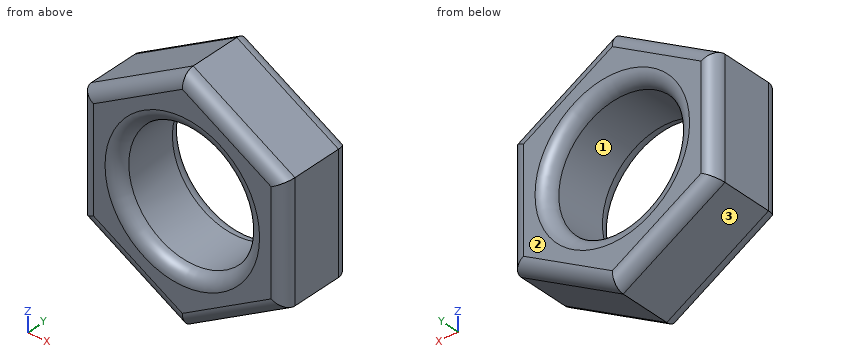
Autodesk Inventor part; units mm, degrees
ref_plane "YZ Plane" through (0, 0, 0) normal (1, 0, 0) x (0, 1, 0)
ref_plane "XZ Plane" through (0, 0, 0) normal (0, 1, 0) x (-1, 0, 0)
ref_plane "XY Plane" through (0, 0, 0) normal (0, 0, 1) x (1, 0, 0)
sketch "Sketch1" plane through (0, 0, 0) normal (0, 1, 0) x (-1, 0, 0)
  line L0 (3.95, -2.2805) -> (0, -4.5611)
  line L1 (0, -4.5611) -> (-3.95, -2.2805)
  line L2 (-3.95, -2.2805) -> (-3.95, 2.2805)
  line L3 (-3.95, 2.2805) -> (0, 4.5611)
  line L4 (0, 4.5611) -> (3.95, 2.2805)
  line L5 (3.95, 2.2805) -> (3.95, -2.2805)
  circle A0 centre (0, 0) radius 2.5
  dimension "d0" = 3.95
  dimension "d1" = 5
extrude "Extrusion1" add sketch "Sketch1" along normal blind 3
fillet "Fillet1" radius 0.5 14 edges at (3.95, 3, 0) (1.975, 3, -3.4208) (-1.975, 3, -3.4208) (-3.95, 3, 0) (-1.975, 3, 3.4208) (1.975, 3, 3.4208) (3.95, 0, 0) (1.975, 0, 3.4208) (-1.975, 0, 3.4208) (-3.95, 0, 0) (-1.975, 0, -3.4208) (1.975, 0, -3.4208) (2.5, 0, 0) (2.5, 3, 0)
thread "Thread1"
properties part number "M5 Nut Silver"
Geometry: final body of the model. Coordinates: model frame, mm. Face numbers are marked on the shaded views. Coordinates: 2 decimals unless noted, no trailing zeros. Order: outer loops, then holes, each group sorted by start corner. A loop starts at its lowest first (then second) coordinate and runs counter-clockwise, first axis right, second up.
Item 1: Section query B-B (y = 0.85). Output: boundary loops of the cut face in (x, z).
Answer:
outline: (-3.95, -2.28) - (0, -4.56) - (3.95, -2.28) - (3.95, 2.28) - (0, 4.56) - (-3.95, 2.28) - close; hole circle Ø5 at (0, 0)
Item 2: Material intervals for line 1 along Z through (x, y) = (-0.25, 1.2); line 2 along Z through (x, y) = (-0.75, 0.25); line 3 along X through (y, z) = (0.5, -1), sorted ascending.
Answer:
line 1: z = -4.42 to -2.49, 2.49 to 4.42
line 2: z = -4.05 to -2.45, 2.45 to 4.05
line 3: x = -3.95 to -2.29, 2.29 to 3.95
Item 3: Section query A-A (z = 0). Output: boundary loops of the cut face in (x, y), then the cut area to 3 significant figures.
Answer:
outline: (-3.95, 0.5) arc R0.5 ccw to (-3.45, 0) - (-3, 0) arc R0.5 ccw to (-2.5, 0.5) - (-2.5, 2.5) arc R0.5 ccw to (-3, 3) - (-3.45, 3) arc R0.5 ccw to (-3.95, 2.5) - close; (2.5, 0.5) arc R0.5 ccw to (3, 0) - (3.45, 0) arc R0.5 ccw to (3.95, 0.5) - (3.95, 2.5) arc R0.5 ccw to (3.45, 3) - (3, 3) arc R0.5 ccw to (2.5, 2.5) - close
area: 8.27 mm2
Item 4: Contact query for a flat-ended pin moving along its axis: P1, Ø1, axis at y = 2, z = -3, coming from the -X side. Output: stop coordinate, or through.
Answer:
P1: stops at x = -3.57
Item 5: Section query C-C (y = 0.2). Output: boundary loops of the cut face in (x, z).
Answer:
outline: (-3.85, -2.22) - (0, -4.45) - (3.85, -2.22) - (3.85, 2.22) - (0, 4.45) - (-3.85, 2.22) - close; hole circle Ø5.2 at (0, 0)
Item 6: Draft query along X for the marked faces 1, 2 and 3. Return one class per face: released by +X, released by -X, zero draft, split by the parting line, or undercut.
Answer:
face 1: undercut
face 2: zero draft
face 3: released by -X
